Design review of the part built by this model. Coordinates are the model's own, in mm. Face numbers are marked on the shaded views. A direction names the side the tool comes from. Give positions to 0.01 mm unless a question says otherwise; leave off trailing zeros. Loops run counter-clockwise (first coordinate to the right, second up) from the corner with the lowest first, then second, coordinate; pieces in that order, holes last. Notation, with made-up numbers: M 22.25,12.5 L 77.25,12.5 A22 ccw 77.25,43.5 Z; hole C -15,56.5 d7. An arc over 180 degrees is marked long. Use a Markdown table: item, result. Add a question column.
(1) Add section A-A, the plane x = 17. Give the boundary of the cut face in (y, z).
(2) Insertion check: pin 1 Ø8.5 at (y, z) = (-18.5, -4) entering from +X; pin 2 Ø3 at (x, y) = (-6, -11.5) entering from -Z; pin 3 Ø1.3 at (x, z) = (17, -12.5) entering from +Y; pin 4 Ø10 at (y, z) = (-17.5, 9) entering from -X. Each pin has a flat end and moves straight along its axis. Give the tip position at first contact, or say it passes through.
(3) Draft analysis for pull direction X (two halves, no side actions). For the marked faces 3, 4, 5 and 6, state which applies: pulls with the +X half, pulls with the -X half, needs draft (parallel to the pull), parting line crosses it, or undercut.
(4) Add section D-D, the plane z = -9.75. State how many separate pieces and enclosed holes the cut face has, then the cut area to 3 significant figures.
(5) Add section C-C, the plane y = -22.5. Give the boundary of the cut face in (x, z).
(6) For the marked faces 1 and 2, list the 3-axis set-ups (+Z, -Z, +X, -X, +Y, -Y) from which the entire face can be reached by the end or side of a thin tool; tool diameter is ignored.
(7) For probe 1 along Z at (x, y) = (0, -14); probe 2 along X at (y, z) = (-13.25, -1); probe 3 along Z at (x, y) = (-8, -18.25), list the stretches that pass through material, from the lowest coordinate up.
(8) Add section B-B, the plane y = -12. Give the boundary of the cut face in (x, z).
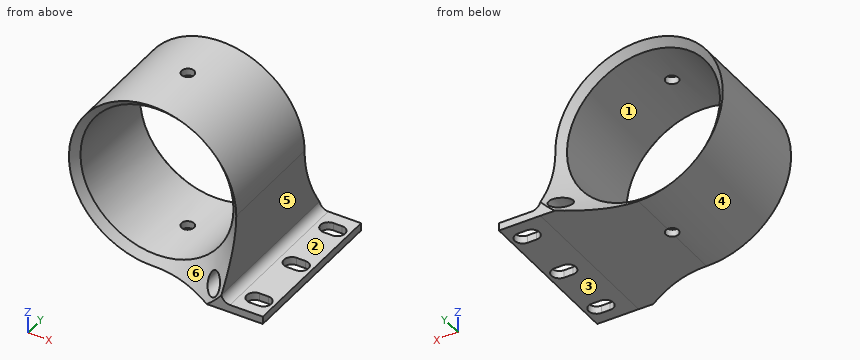
```python
from build123d import *

# Parameters (mm, degrees)
F0_R     = 12.1031
F0_R_2   = 1.397
F1_DEPTH = 25.4
F4_DEPTH = 1.7
F8_R     = 1
F9_DEPTH = 27.8


# Not quite as in the source:
# - a fillet or chamfer that OpenCascade refuses, or shapes differently, is made with other operations: its cross-section is extruded or revolved along the edge and cut away or added


with BuildPart() as f1:
    # F0 (on Front) → F1 (new body)
    with BuildSketch(Plane.XZ):
        with BuildLine():
            ThreePointArc((0.1198459876, -13.2382072509), (9.403486197, -9.3187414184), (13.2387497249, 0))
            ThreePointArc((13.2387497249, 0), (-9.403486197, 9.3187414184), (0.1198459876, -13.2382072509))
        make_face()
        Circle(F0_R, mode=Mode.SUBTRACT)
        with BuildLine():
            Line((13.2387497249, -10.7690971345), (13.2387497249, 0))
            ThreePointArc((13.2387497249, 0), (9.403486197, -9.3187414184), (0.1198459876, -13.2382072509))
            Line((0.1198459876, -13.2382072509), (13.2387497249, -13.1194414571))
            Line((13.2387497249, -13.1194414571), (13.2387497249, -10.7690971345))
        make_face()
        with Locations((11.0441939905, -10.7448566705)):
            Circle(F0_R_2, mode=Mode.SUBTRACT)
        with BuildLine():
            ThreePointArc((14.6132539958, -11.9012827054), (13.7228739986, -11.5817927037), (13.2387497249, -10.7690971345))
            Line((13.2387497249, -10.7690971345), (13.2387497249, -13.1194414571))
            Line((13.2387497249, -13.1194414571), (19.8077764362, -13.1194414571))
            Line((19.8077764362, -13.1194414571), (19.8077764362, -11.9012827054))
            Line((19.8077764362, -11.9012827054), (14.6132539958, -11.9012827054))
        make_face()
    extrude(amount=F1_DEPTH)

    # F3 (on offset) → F4 (cut)
    with BuildSketch(Plane.XY.offset(-13.208)):
        with BuildLine():
            Line((16.5873928428, -4.4316952396), (17.9873928428, -4.4316952396))
            ThreePointArc((17.9873928428, -4.4316952396), (19.2373928428, -3.1816952396), (17.9873928428, -1.9316952396))
            Line((17.9873928428, -1.9316952396), (16.5873928428, -1.9316952396))
            ThreePointArc((16.5873928428, -1.9316952396), (15.3373928428, -3.1816952396), (16.5873928428, -4.4316952396))
        make_face()
        with BuildLine():
            Line((16.5873928428, -13.8912473619), (17.9873928428, -13.8912473619))
            ThreePointArc((17.9873928428, -13.8912473619), (19.2373928428, -12.6412473619), (17.9873928428, -11.3912473619))
            Line((17.9873928428, -11.3912473619), (16.5873928428, -11.3912473619))
            ThreePointArc((16.5873928428, -11.3912473619), (15.3373928428, -12.6412473619), (16.5873928428, -13.8912473619))
        make_face()
        with BuildLine():
            Line((16.5873928428, -23.5218666773), (17.9873928428, -23.5218666773))
            ThreePointArc((17.9873928428, -23.5218666773), (19.2373928428, -22.2718666773), (17.9873928428, -21.0218666773))
            Line((17.9873928428, -21.0218666773), (16.5873928428, -21.0218666773))
            ThreePointArc((16.5873928428, -21.0218666773), (15.3373928428, -22.2718666773), (16.5873928428, -23.5218666773))
        make_face()
    extrude(amount=F4_DEPTH, mode=Mode.SUBTRACT)

    # F5: chamfer of 5 on 1 edges, made by hand

    # F5_s1 → F5_t2 (revolve, cut)
    with BuildSketch(Plane.XY):
        Polygon((17.1031, -25.4), (12.1031, -20.4), (12.1031, -25.4), align=None)
    revolve(axis=Axis((0, -25.4, 0), (0, -1, 0)), mode=Mode.SUBTRACT)

    # F6: chamfer of 5 on 1 edges, made by hand

    # F6_s1 → F6_t2 (revolve, cut)
    with BuildSketch(Plane.XY):
        Polygon((17.1031, 0), (12.1031, -5), (12.1031, 0), align=None)
    revolve(axis=Axis((0, 0, 0), (0, -1, 0)), mode=Mode.SUBTRACT)

    # F8 (on offset) → F9 (cut)
    with BuildSketch(Plane.XY.offset(13.492)):
        with Locations((0, -12.424448505)):
            Circle(F8_R)
    extrude(amount=-F9_DEPTH, mode=Mode.SUBTRACT)


solid = f1.part
```
Established:
| question | item | result |
|---|---|---|
| 1 | outline | M -25.4,-13.12 L -23.52,-13.12 L -23.52,-11.9 L -25.4,-11.9 Z; M -21.02,-13.12 L -13.89,-13.12 L -13.89,-11.9 L -21.02,-11.9 Z; M -11.39,-13.12 L -4.43,-13.12 L -4.43,-11.9 L -11.39,-11.9 Z; M -1.93,-13.12 L 0,-13.12 L 0,-11.9 L -1.93,-11.9 Z |
| 2 | pin 1 | x = 13.24 |
| 2 | pin 2 | z = -12.45 |
| 2 | pin 3 | y = 0 |
| 2 | pin 4 | x = -12.62 |
| 3 | face 3 | needs draft |
| 3 | face 4 | parting line crosses it |
| 3 | face 5 | pulls with the +X half |
| 3 | face 6 | undercut |
| 4 | separate pieces | 3 |
| 4 | enclosed holes | 0 |
| 4 | area | 107 mm^2 |
| 5 | outline | M 5.26,-13.19 L 13.24,-13.12 L 15.36,-13.12 L 15.36,-11.9 L 14.61,-11.9 A1.4 cw 13.24,-10.77 L 13.24,-5.14 A14.2 cw 10.64,-9.41 A1.4 cw long 9.7,-10.38 A14.2 cw Z; M 19.22,-13.12 L 19.81,-13.12 L 19.81,-11.9 L 19.22,-11.9 Z |
| 6 | face 1 | +Y, -Y |
| 6 | face 2 | +Z, +X, +Y, -Y |
| 7 | probe 1 | -13.24 to -12.1, 12.1 to 13.24 |
| 7 | probe 2 | -13.2 to -12.06, 12.06 to 13.24 |
| 7 | probe 3 | -10.55 to -9.08, 9.08 to 10.55 |
| 8 | outline | M -0.91,-13.21 L -0.91,-12.07 A12.1 cw -0.91,12.07 L -0.91,13.21 A13.24 ccw Z; M 0.91,-13.23 L 13.24,-13.12 L 15.51,-13.12 L 15.51,-11.9 L 14.61,-11.9 A1.4 cw 13.24,-10.77 L 13.24,0 A13.24 ccw 0.91,13.21 L 0.91,12.07 A12.1 cw 0.91,-12.07 Z; M 19.06,-13.12 L 19.81,-13.12 L 19.81,-11.9 L 19.06,-11.9 Z; hole C 11.04,-10.74 d2.79 |
